Input: part model. Units: mm. Frame: model coordinates. Coordinates: 2 decimals unless noted, no trailing zeros. Order: outer loops, then holes, each group sorted by start corner. A loop starts at its lowest first (then second) coordinate and runs counter-clockwise, first axis right, second up. Notation, with made-up numbers: (16, -0.5) - (74, -0.5) arc R22 ccw to (74, 34.5) - close; hole circle Ø5 at (-11.75, -38.75). An arc over 180 degrees is marked (long way). One line per question, with ' | ' between items.
from build123d import *

# Parameters (mm, degrees)
F1_DEPTH = 2
F2_R     = 25


with BuildPart() as f1:
    # F0 (on Top) → F1 (new body)
    with BuildSketch(Plane.XY):
        Polygon((-285, -290), (285, -290), (285, 0), (285, 5), (187.5, 5), (187.5, 0), (187.5, -180), (157.5, -180), (157.5, 0), (-157.5, 0), (-157.5, -180), (-187.5, -180), (-187.5, 0), (-187.5, 5), (-285, 5), (-285, 0), align=None)
    extrude(amount=F1_DEPTH)

    # F2
    f2_edges = [f1.edges().sort_by_distance(p)[0] for p in [
        (-157.5, 0, 1),
        (157.5, 0, 1),
    ]]
    fillet(f2_edges, radius=F2_R)


solid = f1.part
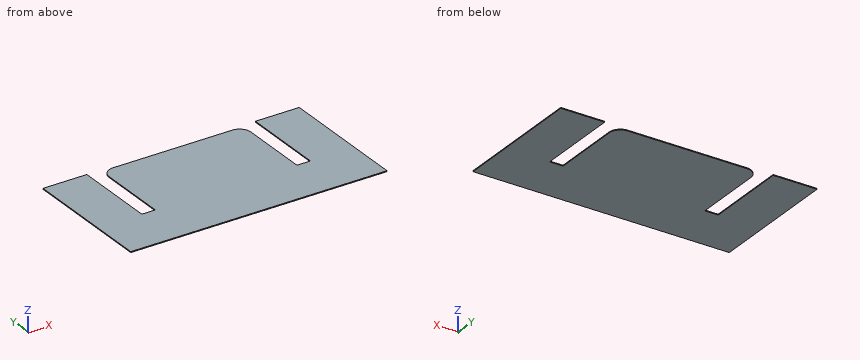
Item 1: Section A-A on y = -169. Return the cut outline in (x, z).
Data:
outline: (-285, 0) - (-187.5, 0) - (-187.5, 2) - (-285, 2) - close; (-157.5, 0) - (157.5, 0) - (157.5, 2) - (-157.5, 2) - close; (187.5, 0) - (285, 0) - (285, 2) - (187.5, 2) - close
Item 2: Section C-C on x = 6.5. Return the cut outline in (y, z), and give its area (3 significant figures).
Data:
outline: (-290, 0) - (0, 0) - (0, 2) - (-290, 2) - close | area: 580 mm^2
Item 3: Ray query, line 1 (X direction, y = -52, z = 1.05); line 2 (Y direction, x = 109, z = 0.75). Return the intervals inside material, ascending.
Data:
line 1: -285 to -187.5, -157.5 to 157.5, 187.5 to 285 | line 2: -290 to 0
Item 4: Section D-D on x = 142.5. Return the cut outline in (y, z).
Data:
outline: (-290, 0) - (-2.09, 0) - (-2.09, 2) - (-290, 2) - close
Item 5: Section B-B on z = 1.4. Return the cut outline in (x, y), and give its area (3 significant figures).
Data:
outline: (-285, -290) - (285, -290) - (285, 5) - (187.5, 5) - (187.5, -180) - (157.5, -180) - (157.5, -25) arc R25 ccw to (132.5, 0) - (-132.5, 0) arc R25 ccw to (-157.5, -25) - (-157.5, -180) - (-187.5, -180) - (-187.5, 5) - (-285, 5) - close | area: 155,000 mm^2
